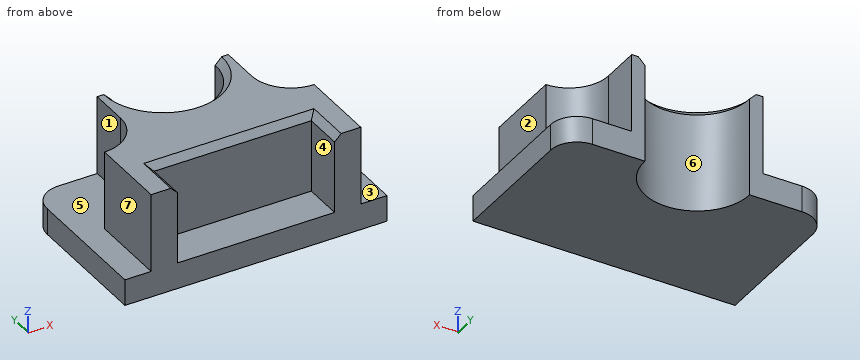
from build123d import *

# Parameters (mm, degrees)
F0_W     = 63.5
F0_H     = 38.1
F1_DEPTH = 6.35
F3_DEPTH = 19.05
F4_DEPTH = 25.4
F5_SIZE  = 1.5875
F7_DEPTH = 25.4
F9_DEPTH = 25.4


with BuildPart() as f1:
    # F0 (on Top) → F1 (new body)
    with BuildSketch(Plane.XY):
        with Locations((31.75, -19.05)):
            Rectangle(F0_W, F0_H)
    extrude(amount=F1_DEPTH)

    # F2 (on face) → F3 (join)
    with BuildSketch(Plane.XY.offset(6.35)):
        with BuildLine():
            Line((6.35, -19.05), (6.35, -38.1))
            Line((6.35, -38.1), (12.7, -38.1))
            Line((12.7, -38.1), (12.7, -28.575))
            Line((12.7, -28.575), (50.8, -28.575))
            Line((50.8, -28.575), (50.8, -38.1))
            Line((50.8, -38.1), (57.15, -38.1))
            Line((57.15, -38.1), (57.15, -19.05))
            ThreePointArc((57.15, -19.05), (50.4148079092, -16.2601920908), (47.625, -9.525))
            Line((47.625, -9.525), (47.625, 0))
            Line((47.625, 0), (44.45, 0))
            ThreePointArc((44.45, 0), (31.75, -12.7), (19.05, 0))
            Line((19.05, 0), (15.875, 0))
            Line((15.875, 0), (15.875, -9.525))
            ThreePointArc((15.875, -9.525), (13.0851920908, -16.2601920908), (6.35, -19.05))
        make_face()
    extrude(amount=F3_DEPTH)

    # F4 (cut): a face of the model
    f4_faces = [f1.faces().sort_by_distance(p)[0] for p in [
        (31.75, -5.390047406, 6.35),
    ]]
    extrude(f4_faces, amount=-F4_DEPTH, mode=Mode.SUBTRACT)

    # F5
    f5_edges = [f1.edges().sort_by_distance(p)[0] for p in [
        (12.7, -33.3375, 25.4),
        (31.75, -28.575, 25.4),
        (50.8, -33.3375, 25.4),
        (31.75, -12.7, 25.4),
    ]]
    chamfer(f5_edges, length=F5_SIZE)

    # F6 (on face) → F7 (cut)
    with BuildSketch(Plane.XY.offset(6.35)):
        with BuildLine():
            Line((6.35, 0), (0, 0))
            Line((0, 0), (0, -6.35))
            ThreePointArc((0, -6.35), (1.8598719395, -1.8598719395), (6.35, 0))
        make_face()
    extrude(amount=-F7_DEPTH, mode=Mode.SUBTRACT)

    # F8 (on face) → F9 (cut)
    with BuildSketch(Plane.XY.offset(6.35)):
        with BuildLine():
            Line((63.5, -6.35), (63.5, 0))
            Line((63.5, 0), (57.15, 0))
            ThreePointArc((57.15, 0), (61.6401280605, -1.8598719395), (63.5, -6.35))
        make_face()
    extrude(amount=-F9_DEPTH, mode=Mode.SUBTRACT)


solid = f1.part
Can you work these out from the model? Positions are in its coordinate system, mm. Face numbers are marked on the shaded views. A direction names the side the tool comes from. Give positions to 0.01 mm unless a question says otherwise; leave off trailing zeros. Order: outer loops, then holes, each group sorted by start corner. A loop starts at its lowest first (then second) coordinate and runs counter-clockwise, first axis right, second up. Notation, with made-up numbers: (6.25, 48) - (41.25, 48) arc R17 ccw to (41.25, 64) - close; hole circle Ø1 at (-18.75, -39.5). An arc over 180 degrees is marked (long way). Write each question's results on one line, items separated by ' | '.
1) On a 3-axis mill with a long thin cutter (end or side, diameter ignored), from which of +Z, -Z, +X, -X, +Y, -Y can I reach the whole of each face in a straight line? I mean the marked faces 1, 2, 3 and 4. Say none if no direction works.
Final values:
face 1: +Z, -X, +Y | face 2: +Z, +X, +Y, -Y | face 3: +Z, +X, +Y | face 4: +Z, -Y
2) If we mould it in two halves opening along X, with no side actions, what happens to the marked faces 5, 6 and 7? For each: pulls with the +X half, pulls with the -X half, needs draft (parallel to the pull), parting line crosses it, or undercut.
Final values:
face 5: needs draft | face 6: undercut | face 7: pulls with the -X half
3) I'm going to push flat-ended pins straight in: pin 1 Ø5 at (x, y) = (32.5, -35) entering from +Z; pin 2 Ø3 at (y, z) = (-5.5, 20) entering from -X (3 decimals); pin 3 Ø6 at (y, z) = (-13, 8.5) entering from +X; pin 4 Ø7.5 at (y, z) = (-6, 14) entering from +X. Where does each tip first touch, or does it pass through?
Final values:
pin 1: stops at z = 6.35 | pin 2: stops at x = 15.875 | pin 3: stops at x = 63.5 | pin 4: stops at x = 47.63
4) Suppose I cut it at D-D, the plane z = 3. Write out the boundary of the cut face in (x, y).
Final values:
outline: (0, -38.1) - (63.5, -38.1) - (63.5, -6.35) arc R6.35 ccw to (57.15, 0) - (44.45, 0) arc R12.7 cw to (19.05, 0) - (6.35, 0) arc R6.35 ccw to (0, -6.35) - close
5) Please list where these lines run through material, in increasing order: line 1 along X through (y, z) = (-32, 22.25); line 2 along Z through (x, y) = (5, -2.5); line 3 along Y through (x, z) = (6.5, 20.5). Write a range as [from, to].
Final values:
line 1: x = [6.35, 12.7], [50.8, 57.15] | line 2: z = [0, 6.35] | line 3: y = [-38.1, -19.05]
6) Suppose I cut it at A-A, the plane y = -34.5. Write out the boundary of the cut face in (x, z).
Final values:
outline: (0, 0) - (63.5, 0) - (63.5, 6.35) - (57.15, 6.35) - (57.15, 25.4) - (52.39, 25.4) - (50.8, 23.81) - (50.8, 6.35) - (12.7, 6.35) - (12.7, 23.81) - (11.11, 25.4) - (6.35, 25.4) - (6.35, 6.35) - (0, 6.35) - close
7) Suppose I cut it at C-C, the plane z = 22.5. Write out the boundary of the cut face in (x, y) (3 decimals), then the cut area to 3 significant figures.
Final values:
outline: (6.35, -38.1) - (12.7, -38.1) - (12.7, -28.575) - (50.8, -28.575) - (50.8, -38.1) - (57.15, -38.1) - (57.15, -19.05) arc R9.525 cw to (47.625, -9.525) - (47.625, 0) - (44.45, 0) arc R12.7 cw to (19.05, 0) - (15.875, 0) - (15.875, -9.525) arc R9.525 cw to (6.35, -19.05) - close | area: 995 mm^2
